The model under review builds one solid part; all positions refer to its coordinate system, in mm. A direction names the side the tool comes from. Round coordinates to 2 decimals unless told otherwise and drop trailing zeros. Write each loop counter-clockwise with the first axis right and the second up, starting at its lowest first coordinate (ties: lowest second). Pieces come first, ordered by that corner, then holes. Notation, with made-up numbers: (69.5, 43) - (100.5, 43) arc R26 ccw to (100.5, 77) - close; hole circle Ø1 at (37.5, 5). An arc over 180 degrees is marked (long way). Use one line per item in the form item = value.
from build123d import *
from build123d.topology import SkipClean

# Parameters (mm, degrees)
SKETCH1_R                      = 1.5
BOSS_EXTRUDE1_DEPTH            = 5
CUT_EXTRUDE1_DEPTH             = 17.293347298
CUT_EXTRUDE1_DEPTH_BACK        = 17.293347298
SKETCH2_W                      = 6
SKETCH2_H                      = 12
SKETCH5_W                      = 7.867189124
SKETCH5_H                      = 6
BOSS_EXTRUDE2_DEPTH            = 10
SKETCH6_R                      = 1
SKETCH6_R_2                    = 1.625
BOSS_EXTRUDE3_DEPTH            = 5
BOSS_EXTRUDE4_DEPTH            = 2.5
BOSS_EXTRUDE4_DEPTH_BACK       = 7.5
SKETCH7_R                      = 1
CUT_EXTRUDE2_REACH             = 54.5
SKETCH8_W                      = 6
SKETCH8_H                      = 9
CUT_EXTRUDE2_DIRECTION_2_DEPTH = 53.5


with BuildPart() as part:
    # Sketch1 → Boss-Extrude1 (new, symmetric)
    with BuildSketch(Plane(origin=(0, 0, 0), x_dir=(0, 0, -1), z_dir=(1, 0, 0))):
        with BuildLine():
            Line((3.933594562, 0), (3.933594562, -15))
            Line((3.933594562, -15), (-3.933594562, -15))
            Line((-3.933594562, -15), (-3.933594562, 0))
            ThreePointArc((-3.933594562, 0), (0, 3.933594562), (3.933594562, 0))
        make_face()
        Circle(SKETCH1_R, mode=Mode.SUBTRACT)
    extrude(amount=BOSS_EXTRUDE1_DEPTH, both=True)

    # Sketch2 → Cut-Extrude1 (cut, two sides: drawn at the far end of the back side and taken through both)
    with BuildSketch(Plane.XY.offset(-CUT_EXTRUDE1_DEPTH_BACK)):
        with Locations((0, -2.066405438)):
            Rectangle(SKETCH2_W, SKETCH2_H)
    extrude(amount=CUT_EXTRUDE1_DEPTH + CUT_EXTRUDE1_DEPTH_BACK, mode=Mode.SUBTRACT)

    # Sketch5 → Boss-Extrude2 (add)
    with BuildSketch(Plane.ZY.offset(5)):
        with Locations((0, -12)):
            Rectangle(SKETCH5_W, SKETCH5_H)
    extrude(amount=BOSS_EXTRUDE2_DEPTH)

    # Sketch6 → Boss-Extrude3 (add)
    with BuildSketch(Plane.ZY.offset(15)):
        with BuildLine():
            Line((23.199216315, -9), (-6.066405438, -9))
            Line((-6.066405438, -9), (-6.066405438, -2.25))
            ThreePointArc((-6.066405438, -2.25), (-10, 1.683594562), (-13.933594562, -2.25))
            Line((-13.933594562, -2.25), (-13.933594562, -6.757725184))
            Line((-13.933594562, -6.757725184), (-13.933594562, -15))
            Line((-13.933594562, -15), (31.066405438, -15))
            Line((31.066405438, -15), (31.066405438, -6.757725184))
            Line((31.066405438, -6.757725184), (31.066405438, -2.25))
            ThreePointArc((31.066405438, -2.25), (27.132810876, 1.683594562), (23.199216315, -2.25))
            Line((23.199216315, -2.25), (23.199216315, -9))
        make_face()
        with Locations((-10, -2.25)):
            Circle(SKETCH6_R, mode=Mode.SUBTRACT)
        with Locations((27.132810876, -2.25)):
            Circle(SKETCH6_R_2, mode=Mode.SUBTRACT)
    extrude(amount=BOSS_EXTRUDE3_DEPTH)

    # Sketch7 → Boss-Extrude4 (add, two sides: drawn at the far end of the back side and taken through both)
    with SkipClean():  # the faces are left unmerged after this step: merging them gives an invalid solid
        with BuildSketch(Plane.ZY.offset(20).offset(-BOSS_EXTRUDE4_DEPTH_BACK)):
            with BuildLine():
                Line((-13.933594562, -15), (-13.933594562, -2.25))
                ThreePointArc((-13.933594562, -2.25), (-10, 1.683594562), (-6.066405438, -2.25))
                Line((-6.066405438, -2.25), (-6.066405438, -15))
                Line((-6.066405438, -15), (-13.933594562, -15))
            make_face()
            with Locations((-10, -2.25)):
                Circle(SKETCH7_R, mode=Mode.SUBTRACT)
        extrude(amount=BOSS_EXTRUDE4_DEPTH + BOSS_EXTRUDE4_DEPTH_BACK)
    add(part.part.scale(1), mode=Mode.REPLACE)  # the faces are merged on a copy

    # Sketch8 → Cut-Extrude2 (cut, up to next)
    with BuildSketch(Plane(origin=(0, 0, -13.933594562), x_dir=(-1, 0, 0), z_dir=(0, 0, -1)), mode=Mode.PRIVATE) as cut_extrude2_sk1:
        with Locations((17.5, -2.816405438)):
            Rectangle(SKETCH8_W, SKETCH8_H)
    cut_extrude2_tool1 = extrude(cut_extrude2_sk1.sketch, amount=-CUT_EXTRUDE2_REACH, mode=Mode.PRIVATE) & part.part
    add(cut_extrude2_tool1.solids().sort_by_distance((-17.5, -2.816405, -13.933595))[0], mode=Mode.SUBTRACT)

    # Sketch8 → Cut-Extrude2 direction 2 (cut)
    with BuildSketch(Plane(origin=(0, 0, -13.933594562), x_dir=(-1, 0, 0), z_dir=(0, 0, -1))):
        with Locations((17.5, -2.816405438)):
            Rectangle(SKETCH8_W, SKETCH8_H)
    extrude(amount=CUT_EXTRUDE2_DIRECTION_2_DEPTH, mode=Mode.SUBTRACT)


solid = part.part
(1) The part is to be moulded in two halves that separate along Z. For faces 1 (the flat face through (-12.5, -7, -10)), 2 (the cylindrical face through (4.014, 3.933, 0.086)), 3 (the cylindrical face through (-4.01, 0.07, 1.5)), say which applies: +Z half, -Z half, draft (parallel to the pull), parting line (faces both ways), or undercut.
Geometry results:
face_1 = draft
face_2 = parting line
face_3 = undercut
(2) Machinability: for faces 4 (the flat face through (3, -2, 0)), 5 (the flat face through (-17.4, -8.5, -6.066)), 6 (the flat face through (-17, -6, 23.199)), 7 (the flat face through (-15, -12, -5)), which of the approach directions +Z, -Z, +X, -X, +Y, -Y give a long, thin tool a straight path to every point of the face, cutting with its end or side? Answer none if there is none.
Geometry results:
face_4 = +Z, -Z, +Y
face_5 = +Y
face_6 = +X, -X, +Y
face_7 = +X, +Y, -Y
(3) To check wall thickness, follow L1, parallel to Y at x = -13.55, z = -10; L2, parallel to Z at x = -21.05, y = -2.25; L3, parallel to X at y = -5.75, z = 1. State the ranges of each line that lie inside material, in increasing order.
Geometry results:
L1 = -15 to -3.25, -1.25 to 1.68
L2 = -13.93 to -11, -9 to -6.07
L3 = -5 to -3, 3 to 5
(4) Add section C-C on x = -4. Write out the cut boundary in (y, z).
Geometry results:
outline = (-15, -3.93) - (0, -3.93) arc R3.93 ccw to (0, 3.93) - (-15, 3.93) - close; hole circle Ø3 at (0, 0)
(5) Add section A-A on z = -10. Write out the cut boundary in (x, y), then the cut area to 3 significant figures.
Geometry results:
outline = (-22.5, -15) - (-12.5, -15) - (-12.5, -3.25) - (-14.5, -3.25) - (-14.5, -7.32) - (-20.5, -7.32) - (-20.5, -3.25) - (-22.5, -3.25) - close; (-22.5, -1.25) - (-20.5, -1.25) - (-20.5, 1.68) - (-22.5, 1.68) - close; (-14.5, -1.25) - (-12.5, -1.25) - (-12.5, 1.68) - (-14.5, 1.68) - close
area = 105 mm2
(6) Add section D-D on y = -11. Write out the cut boundary in (x, z), then the cut area to 3 significant figures.
Geometry results:
outline = (-22.5, -13.93) - (-12.5, -13.93) - (-12.5, -6.07) - (-15, -6.07) - (-15, -3.93) - (5, -3.93) - (5, 3.93) - (-15, 3.93) - (-15, 31.07) - (-20, 31.07) - (-20, -6.07) - (-22.5, -6.07) - close
area = 422 mm2
(7) Add section B-B on y = -5.75. Write out the cut boundary in (x, z).
Geometry results:
outline = (-22.5, -13.93) - (-20.5, -13.93) - (-20.5, -6.07) - (-22.5, -6.07) - close; (-20, 23.2) - (-15, 23.2) - (-15, 31.07) - (-20, 31.07) - close; (-14.5, -13.93) - (-12.5, -13.93) - (-12.5, -6.07) - (-14.5, -6.07) - close; (-5, -3.93) - (-3, -3.93) - (-3, 3.93) - (-5, 3.93) - close; (3, -3.93) - (5, -3.93) - (5, 3.93) - (3, 3.93) - close
(8) Insertion check: P1, Ø2.5, axis at y = -4.5, z = -0.5, coming from the -X side; P2, Ø2.5, axis at y = -3.5, z = -10.5, coming from the +X side; P3, Ø2, axis at y = -9.5, z = 11.5, coming from the +X side. Each pin has a flat end and moves straight along its axis. Give the tip position at first contact, or say it passes through.
Geometry results:
P1 = -5
P2 = -12.5
P3 = -15
